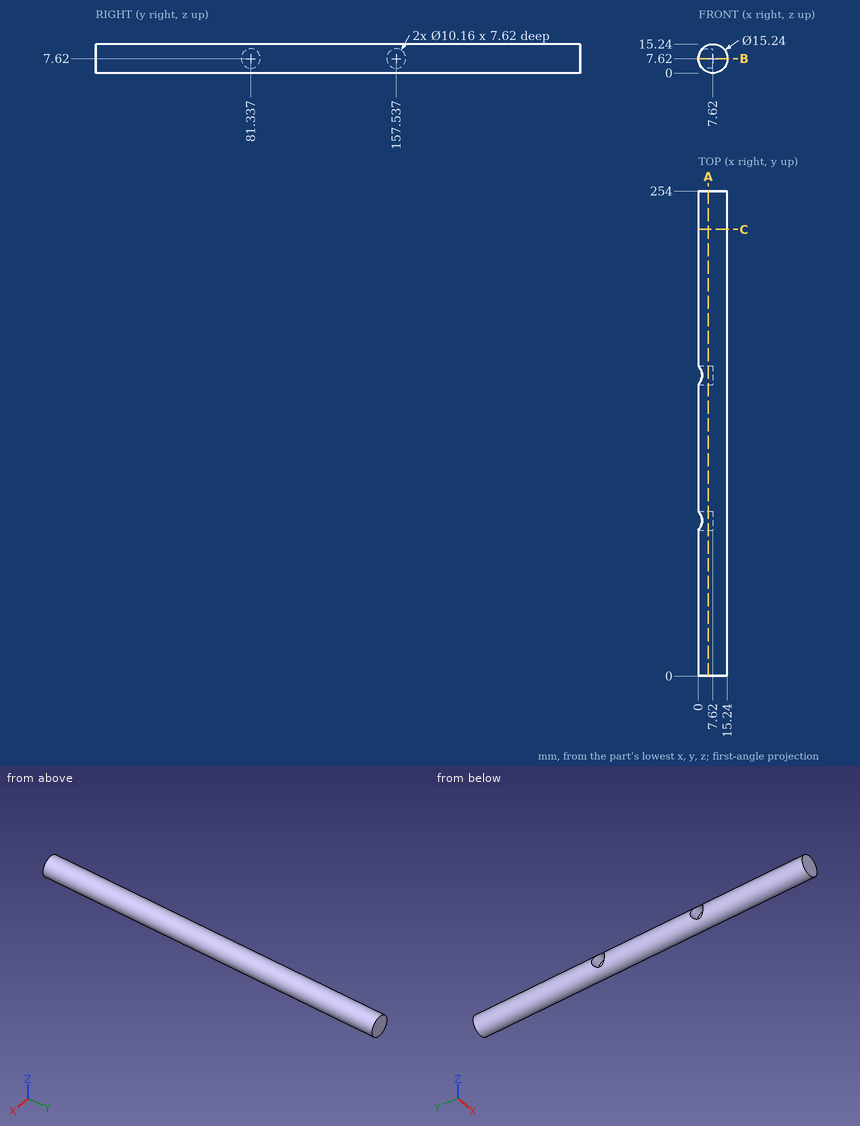
The drawing under review shows one solid part. Ordinate dimensions are in mm from its lowest x, y, z. Round coordinates to 2 decimals unless told otherwise and drop trailing zeros. Write each loop counter-clockwise with the first axis right and the second up, starting at its lowest first coordinate (ties: lowest second). Pieces come first, ordered by that corner, then holes. Notation, with made-up numbers: (-6, 28) -> (33, 28) arc R18 ccw to (33, 38) -> close; hole circle Ø6 at (39.5, 77.25). An arc over 180 degrees is marked (long way). One line per question, with ' | ' between items. Start each with the question number.
(1) Insertion check: P1, Ø5, axis at y = 83.5, z = 8.5, coming from the -X side; P2, Ø1.5, axis at y = 36.5, z = 3, coming from the +X side; P3, Ø3, axis at x = 13, y = 206.5, coming from the +Z side. Each pin has a flat end and moves straight along its axis. Give the tip position at first contact, or say it passes through.
(2) Add section A-A, the plane x = 5.25. Write out the cut boundary in (y, z), plus the area to 3 significant figures.
(3) Add section B-B, the plane z = 7.62. Write out the cut boundary in (x, y), plus the area to 3 significant figures.
(4) Add section C-C, the plane y = 234. Write out the cut boundary in (x, z), plus the area to 3 significant figures.
(5) For line 1 along Y through (x, z) = (2.25, 7.62); line 2 along Y through (x, z) = (4.5, 10) (1 decimal); line 3 along X through (y, z) = (116.5, 8.25), list the stretches that pass through material, from the lowest coordinate up. Write a range as from..to.
Answer list:
1) P1: x = 7.62 | P2: x = 14.18 | P3: z = 14.18
2) outline: (0, 0.38) -> (254, 0.38) -> (254, 14.86) -> (0, 14.86) -> close; hole circle Ø10.16 at (81.34, 7.62); hole circle Ø10.16 at (157.54, 7.62) | area: 3,520 mm²
3) outline: (0, 0) -> (15.24, 0) -> (15.24, 254) -> (0, 254) -> (0, 162.62) -> (7.62, 162.62) -> (7.62, 152.46) -> (0, 152.46) -> (0, 86.42) -> (7.62, 86.42) -> (7.62, 76.26) -> (0, 76.26) -> close | area: 3,720 mm²
4) outline: circle Ø15.24 at (7.62, 7.62) | area: 182 mm²
5) line 1: 0..76.26, 86.42..152.46, 162.62..254 | line 2: 0..76.8, 85.8..153, 162..254 | line 3: 0.03..15.21
